The model under review builds one solid part; all positions refer to its coordinate system, in mm. A direction names the side the tool comes from. Round coordinates to 2 decimals unless told otherwise and drop trailing zeros. Order: outer loops, then holes, each group sorted by start corner. A loop starts at its lowest first (then second) coordinate and runs counter-clockwise, first axis right, second up.
```python
from build123d import *

# Parameters (mm, degrees)
SKETCH012_AS_DRAWN_R                 = 62
EXTRUDE005_DEPTH                     = 50
EXTRUDE005_ONTO_SKETCH012_ROLL_ANGLE = 90
SKETCH013_R                          = 57
POCKET003_DEPTH                      = 2
SKETCH014_R                          = 51
POCKET004_DEPTH                      = 8
SKETCH015_R                          = 47
POCKET005_DEPTH                      = 26
SKETCH016_R                          = 58
POCKET006_DEPTH                      = 2
SKETCH017_R                          = 51
POCKET007_DEPTH                      = 2
POCKET008_DEPTH                      = 9
POCKET009_DEPTH                      = 5
POCKET010_DEPTH                      = 8
SKETCH022_R                          = 4
POCKET011_DEPTH                      = 38.001


with BuildPart() as part:
    # Sketch012 as drawn → Extrude005 (new)
    with BuildSketch(Plane.XY):
        Circle(SKETCH012_AS_DRAWN_R)
    extrude(amount=-EXTRUDE005_DEPTH)


with BuildPart() as part_1:
    # Extrude005 onto Sketch012 roll: moved
    add(part.part.rotate(Axis((0, 0, 0), (1, 0, 0)), EXTRUDE005_ONTO_SKETCH012_ROLL_ANGLE))


with BuildPart() as part_2:
    # Extrude005 onto Sketch012 placement: moved
    add(part_1.part)

    # Sketch013 → Pocket003 (cut)
    with BuildSketch(Plane.XZ):
        Circle(SKETCH013_R)
    extrude(amount=-POCKET003_DEPTH, mode=Mode.SUBTRACT)

    # Sketch014 → Pocket004 (cut)
    with BuildSketch(Plane.XZ.offset(-2)):
        Circle(SKETCH014_R)
    extrude(amount=-POCKET004_DEPTH, mode=Mode.SUBTRACT)

    # Sketch015 → Pocket005 (cut)
    with BuildSketch(Plane.XZ.offset(-10)):
        Circle(SKETCH015_R)
    extrude(amount=-POCKET005_DEPTH, mode=Mode.SUBTRACT)

    # Sketch016 → Pocket006 (cut)
    with BuildSketch(Plane(origin=(0, 50, 0), x_dir=(-1, 0, 0), z_dir=(0, 1, 0))):
        Circle(SKETCH016_R)
    extrude(amount=-POCKET006_DEPTH, mode=Mode.SUBTRACT)

    # Sketch017 → Pocket007 (cut)
    with BuildSketch(Plane(origin=(0, 48, 0), x_dir=(-1, 0, 0), z_dir=(0, 1, 0))):
        Circle(SKETCH017_R)
    extrude(amount=-POCKET007_DEPTH, mode=Mode.SUBTRACT)

    # Sketch019 → Pocket008 (cut)
    with BuildSketch(Plane(origin=(0, 46, 0), x_dir=(-1, 0, 0), z_dir=(0, 1, 0))):
        with BuildLine():
            ThreePointArc((50.641544, 0.353553), (35.708892, 35.708892), (0.353553, 50.641544))
            Line((0.353553, 24.353553), (0.353553, 50.641544))
            ThreePointArc((24.353553, 0.353553), (17.324116, 17.324116), (0.353553, 24.353553))
            Line((24.353553, 0.353553), (50.641544, 0.353553))
        make_face()
        with BuildLine():
            ThreePointArc((0.353553, -24.353553), (17.324116, -17.324116), (24.353553, -0.353553))
            Line((24.353553, -0.353553), (51.353553, -0.353553))
            ThreePointArc((0.353553, -51.353553), (36.415999, -36.415999), (51.353553, -0.353553))
            Line((0.353553, -24.353553), (0.353553, -51.353553))
        make_face()
        with BuildLine():
            ThreePointArc((-24.353553, -0.353553), (-17.324116, -17.324116), (-0.353553, -24.353553))
            Line((-0.353553, -24.353553), (-0.353553, -51.353553))
            ThreePointArc((-51.353553, -0.353553), (-36.415999, -36.415999), (-0.353553, -51.353553))
            Line((-24.353553, -0.353553), (-51.353553, -0.353553))
        make_face()
        with BuildLine():
            ThreePointArc((-0.353553, 24.353553), (-17.324116, 17.324116), (-24.353553, 0.353553))
            Line((-24.353553, 0.353553), (-51.353553, 0.353553))
            ThreePointArc((-0.353553, 51.353553), (-36.415999, 36.415999), (-51.353553, 0.353553))
            Line((-0.353553, 24.353553), (-0.353553, 51.353553))
        make_face()
    extrude(amount=-POCKET008_DEPTH, mode=Mode.SUBTRACT)

    # Sketch020 → Pocket009 (cut)
    with BuildSketch(Plane(origin=(0, 46, 0), x_dir=(-1, 0, 0), z_dir=(0, 1, 0))):
        with BuildLine():
            Line((-24.353553, 0.353553), (-17.35351, 0.353553))
            ThreePointArc((-0.353553, 17.353553), (-12.374341, 12.374353), (-17.35351, 0.353553))
            Line((-0.353553, 17.353553), (-0.353553, 24.353553))
            Line((-0.353553, 24.353553), (-24.353553, 24.353553))
            Line((-24.353553, 24.353553), (-24.353553, 0.353553))
        make_face()
        with BuildLine():
            Line((24.353553, 0.353553), (17.353553, 0.353553))
            ThreePointArc((17.353553, 0.353553), (12.374369, 12.374369), (0.353553, 17.353553))
            Line((0.353553, 17.353553), (0.353553, 24.353553))
            Line((0.353553, 24.353553), (24.353553, 24.353553))
            Line((24.353553, 24.353553), (24.353553, 0.353553))
        make_face()
        with BuildLine():
            Line((-0.353553, -24.353553), (-24.353553, -24.353553))
            Line((-24.353553, -24.353553), (-24.353553, -0.353553))
            Line((-24.353553, -0.353553), (-17.35351, -0.353553))
            ThreePointArc((-17.35351, -0.353553), (-12.374341, -12.374353), (-0.353553, -17.353553))
            Line((-0.353553, -17.353553), (-0.353553, -24.353553))
        make_face()
        with BuildLine():
            Line((0.353553, -24.353553), (24.353553, -24.353553))
            Line((24.353553, -24.353553), (24.353553, -0.353553))
            Line((24.353553, -0.353553), (17.353553, -0.353553))
            ThreePointArc((0.353553, -17.353553), (12.374369, -12.374369), (17.353553, -0.353553))
            Line((0.353553, -17.353553), (0.353553, -24.353553))
        make_face()
    extrude(amount=-POCKET009_DEPTH, mode=Mode.SUBTRACT)

    # Sketch021 → Pocket010 (cut)
    with BuildSketch(Plane(origin=(0, 46, 0), x_dir=(-1, 0, 0), z_dir=(0, 1, 0))):
        Polygon((6, -10.392305), (12, 0), (6, 10.392305), (-6, 10.392305), (-12, 0), (-6, -10.392305), align=None)
    extrude(amount=-POCKET010_DEPTH, mode=Mode.SUBTRACT)

    # Sketch022 → Pocket011 (cut, through all)
    with BuildSketch(Plane(origin=(0, 38, 0), x_dir=(-1, 0, 0), z_dir=(0, 1, 0))):
        Circle(SKETCH022_R)
    extrude(amount=-POCKET011_DEPTH, mode=Mode.SUBTRACT)


solid = part_2.part
```
(1) Insertion check: pin 1 (3 mm diameter, centred on y = 20.5, z = -16, fed in from -X); pin 2 (3 mm diameter, centred on x = 37.5, y = 7, fed in from -Z); pin 3 (4.5 mm diameter, centred on x = -28.5, y = 43, fed in from +Z). Each pin has a flat end and moves straight along its axis. Give the tip position at first contact, or say it passes through.
Data:
pin 1: stops at x = -60.28
pin 2: stops at z = -50.48
pin 3: stops at z = 56.17
(2) For faces 3 (the cylindrical face through (-11.056, 5.944, -49.787)), 4 (the flat face through (-12, 41, -15)), list the 3-axis set-ups (+Z, -Z, +X, -X, +Y, -Y) from which the entire face can be reached by the end or side of a thin tool; tool diameter is ignored.
Data:
face 3: -Y
face 4: +Y
(3) Draft analysis for pull direction X (two halves, no side actions). For faces 1 (the flat face through (50.23, 0, -27.27)), 2 (the flat face through (0.354, 42, -34)), state which applies: pulls with the +X half, pulls with the -X half, needs draft (parallel to the pull), parting line crosses it, or undercut.
Data:
face 1: needs draft
face 2: undercut
(4) To check wall thickness, follow probe 1 along X at (y, z) = (43, 45); probe 2 along Z at (x, y) = (0, 36.75); probe 3 along Y at (x, z) = (54, 13). State the ranges of each line that lie inside material, in increasing order.
Data:
probe 1: x = -42.65 to -22.97, -0.35 to 0.35, 25.01 to 42.65
probe 2: z = -62 to -4, 4 to 62
probe 3: y = 2 to 48
(5) Consider section D-D (y = 3.5). Write out the cut boundary in (x, z), and give its area (4 significant figures).
Data:
outline: circle Ø124 at (0, 0); hole circle Ø102 at (0, 0)
area: 3,905 mm2
(6) Consider section A-A (y = 26.5). Write out the cut boundary in (x, z), and give its area (3 significant figures).
Data:
outline: circle Ø124 at (0, 0); hole circle Ø94 at (0, 0)
area: 5,140 mm2
